from build123d import *

# Parameters (mm, degrees)
F2_W          = 125
F2_H          = 25
F3_DEPTH      = 8
F4_DEPTH      = 25
F6_DEPTH      = 1
F6_DEPTH_BACK = 25
F8_DEPTH      = 5
F10_DEPTH     = 25


with BuildPart() as f3:
    # F2 (on offset) → F3 (new body)
    with BuildSketch(Plane.XY.offset(-3)):
        with Locations((0, 94.5)):
            Rectangle(F2_W, F2_H)
        Polygon((-62.5, 82), (-62.5, 107), (-76.9337567297, 82), align=None)
        Polygon((76.9337567297, 82), (62.5, 107), (62.5, 82), align=None)
    extrude(amount=F3_DEPTH)

    # F0 (on Top) → F4 (cut)
    with BuildSketch(Plane.XY):
        with BuildLine():
            Line((-90.4997997897, 42.5415824579), (90.4997997897, 42.5415824579))
            ThreePointArc((90.4997997897, 42.5415824579), (0, 100), (-90.4997997897, 42.5415824579))
        make_face()
    extrude(amount=F4_DEPTH, mode=Mode.SUBTRACT)

    # F5 (on Top) → F6 (cut, two sides)
    with BuildSketch(Plane.XY) as f6_sk:
        with BuildLine():
            Line((4, 82), (4, 84.8831560302))
            ThreePointArc((4, 84.8831560302), (0, 103), (-4, 84.8831560302))
            Line((-4, 84.8831560302), (-4, 82))
            Line((-4, 82), (4, 82))
        make_face()
    extrude(amount=-F6_DEPTH, mode=Mode.SUBTRACT)
    extrude(f6_sk.sketch, amount=F6_DEPTH_BACK, mode=Mode.SUBTRACT)

    # F7 (on face) → F8 (cut)
    with BuildSketch(Plane.XY.offset(5)):
        with BuildLine():
            Line((62.5, 207), (58.7661641518, 207))
            ThreePointArc((58.7661641518, 207), (49.6095920415, 196.0748240465), (51.8682665386, 182))
            Line((51.8682665386, 182), (76.9337567297, 182))
            Line((76.9337567297, 182), (62.5, 207))
        make_face()
        with BuildLine():
            ThreePointArc((-51.8682665386, 182), (-49.6095920415, 196.0748240465), (-58.7661641518, 207))
            Line((-58.7661641518, 207), (-62.5, 207))
            Line((-62.5, 207), (-76.9337567297, 182))
            Line((-76.9337567297, 182), (-51.8682665386, 182))
        make_face()
    extrude(amount=-F8_DEPTH, mode=Mode.SUBTRACT)

    # F9 (on offset) → F10 (cut)
    with BuildSketch(Plane.XY.offset(-3)):
        with BuildLine():
            Line((55.8554306626, 86), (66.1950417228, 86))
            ThreePointArc((66.1950417228, 86), (68.3950417228, 88.2), (66.1950417228, 90.4))
            Line((66.1950417228, 90.4), (55.8554306626, 90.4))
            Line((55.8554306626, 90.4), (45.5158196025, 90.4))
            ThreePointArc((45.5158196025, 90.4), (43.3158196025, 88.2), (45.5158196025, 86))
            Line((45.5158196025, 86), (55.8554306626, 86))
        make_face()
        with BuildLine():
            ThreePointArc((-66.1950417228, 90.4), (-68.3950417228, 88.2), (-66.1950417228, 86))
            Line((-66.1950417228, 86), (-55.8554306626, 86))
            Line((-55.8554306626, 86), (-45.5158196025, 86))
            ThreePointArc((-45.5158196025, 86), (-43.3158196025, 88.2), (-45.5158196025, 90.4))
            Line((-45.5158196025, 90.4), (-55.8554306626, 90.4))
            Line((-55.8554306626, 90.4), (-66.1950417228, 90.4))
        make_face()
    extrude(amount=F10_DEPTH, mode=Mode.SUBTRACT)


solid = f3.part
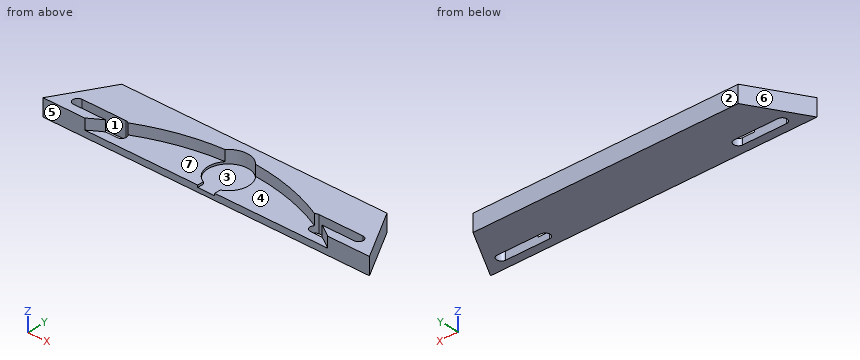
Check sheet for the modelled part. Datum: model origin and axes. Units: mm. Face numbers are marked on the shaded views. A direction names the side the tool comes from. Round coordinates to 2 decimals unless told otherwise and drop trailing zeros. Write each loop counter-clockwise with the first axis right and the second up, starting at its lowest first coordinate (ties: lowest second). Pieces come first, ordered by that corner, then holes. Notation, with made-up numbers: (22.5, -33.75) - (81.5, -33.75) arc R28 cw to (81.5, 2.25) - close; hole circle Ø10 at (-29, 81). An arc over 180 degrees is marked (long way). Return JSON: item names as keys, results as strings.
Q1. Draft check along X on the marked faces 5, 6 and 7. Enter one of: released by +X, released by -X, zero draft, split by the parting line, or undercut.
Returned:
{"face 5": "zero draft", "face 6": "released by -X", "face 7": "undercut"}
Q2. Cross-section at B-B (y = 88.2). Record the boundary of the cut face in (x, z), then the cut area to 3 significant figures.
Returned:
{"outline": "(-73.35, -3) - (-68.4, -3) - (-68.4, 5) - (-73.35, 5) - close; (-43.32, -3) - (43.32, -3) - (43.32, 0) - (7.88, 0) - (7.88, -1) - (-7.88, -1) - (-7.88, 0) - (-43.32, 0) - close; (68.4, -3) - (73.35, -3) - (73.35, 5) - (68.4, 5) - close", "area": "323 mm²"}
Q3. Access from +Z, -Z, +X, -X, +Y, -Y to the whole of each face (thin tool, end or side, straight path). Record for the marked faces 1, 2, 3 and 4.
Returned:
{"face 1": "+Z, -Z", "face 2": "+Z, -Z, +X, -X, +Y", "face 3": "+Z", "face 4": "+Z, -Y"}
Q4. Depth check by flat-ended pin: P1, Ø10, axis at x = 11, y = 88.5, coming from the +Z side; P2, Ø4, axis at y = 91, z = 0.5, coming from the -X side; P3, Ø1.5, axis at y = 101, z = -1.5, coming from the +X side. Enter the tip coordinate at first touch or a pass-through.
Returned:
{"P1": "stops at z = 0", "P2": "stops at x = -72.89", "P3": "stops at x = 66.4"}
Q5. Cross-section at A-A (x = 48.5). Record the boundary of the cut face in (y, z), then the cut area to 3 significant figures.
Returned:
{"outline": "(82, -3) - (86, -3) - (86, 0) - (82, 0) - close; (90.4, -3) - (107, -3) - (107, 5) - (90.4, 5) - close", "area": "145 mm²"}
Q6. Cross-section at D-D (y = 96). Record the boundary of the cut face in (x, z), then the cut area to 3 significant figures.
Returned:
{"outline": "(-68.85, -3) - (68.85, -3) - (68.85, 5) - (28, 5) - (28, 0) - (9.17, 0) - (9.17, -1) - (-9.17, -1) - (-9.17, 0) - (-28, 0) - (-28, 5) - (-68.85, 5) - close", "area": "803 mm²"}
Q7. Cross-section at C-C (z = 2). Record the boundary of the cut face in (x, y).
Returned:
{"outline": "(-76.93, 82) - (-57.24, 82) arc R100 cw to (-51.03, 86) - (-66.2, 86) arc R2.2 cw to (-66.2, 90.4) - (-45.52, 90.4) arc R2.2 cw to (-44, 89.8) arc R100 cw to (-7.16, 99.74) arc R9.5 cw to (7.16, 99.74) arc R100 cw to (44, 89.8) arc R2.2 cw to (45.52, 90.4) - (66.2, 90.4) arc R2.2 cw to (66.2, 86) - (51.03, 86) arc R100 cw to (57.24, 82) - (76.93, 82) - (62.5, 107) - (-62.5, 107) - close"}
Q8. Scan lines: L1, parallel to Y at x = -56, z = -2.5; L2, parallel to Z at x = -24, y = 85.5; L3, parallel to X at y = 100.5, z = 3. Record each from-to range of solid material in increasing order. Write a range as from..to.
Returned:
{"L1": "y = 82..86, 90.4..107", "L2": "z = -3..0", "L3": "x = -66.25..-6.42, 6.42..66.25"}
